Build history of the part. All positions in model axes, mm. Face numbers are marked on the shaded views. Give positions to 0.01 mm unless a question says otherwise; leave off trailing zeros. Order: outer loops, then holes, each group sorted by start corner. A loop starts at its lowest first (then second) coordinate and runs counter-clockwise, first axis right, second up. Notation, with made-up numbers: (8.25, 3.5) - (62.25, 3.5) arc R22 ccw to (62.25, 29.5) - close; hole circle Ø10 at (42, 25). An arc over 180 degrees is marked (long way). One line per item, written item: value.
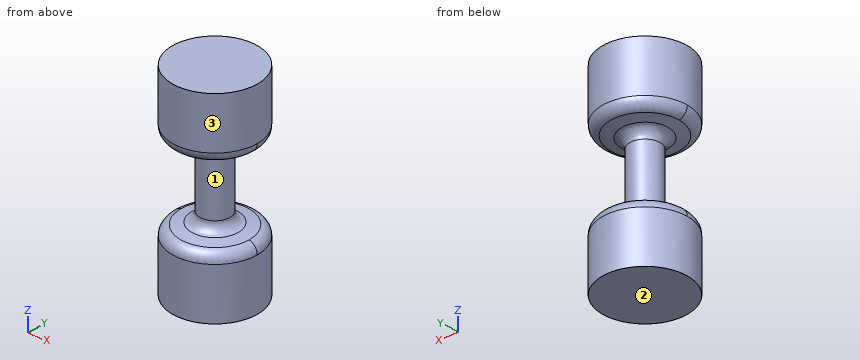
```python
from build123d import *

# Parameters (mm, degrees)
BOSS_EXTRUDE1_DEPTH      = 20
BOSS_EXTRUDE1_DEPTH_BACK = 20
SKETCH1_R                = 8.5
FILLET1_R                = 2


# Read off the part's stored shape, not the designer's step: Shell1
with BuildPart() as part:
    # Sketch1 → Boss-Extrude1 (new, two sides: drawn at the far end of the back side and taken through both)
    with BuildSketch(Plane.XY.offset(-BOSS_EXTRUDE1_DEPTH_BACK)):
        Circle(SKETCH1_R)
    extrude(amount=BOSS_EXTRUDE1_DEPTH + BOSS_EXTRUDE1_DEPTH_BACK)

    # Sketch2 → Cut-Revolve1 (revolve, cut)
    with BuildSketch(Plane(origin=(0, 0, 0), x_dir=(0, 0, -1), z_dir=(1, 0, 0)), mode=Mode.PRIVATE) as cut_revolve1_sk:
        Polygon((-8, 8.5), (8, 8.5), (7, 3), (-7, 3), align=None)
    revolve(cut_revolve1_sk.sketch.rotate(Axis((0, 0, -22), (0, 0, 1)), 90), axis=Axis((0, 0, -22), (0, 0, 1)), mode=Mode.SUBTRACT)

    # Shell1 outline → Shell1 (revolve, cut)
    with BuildSketch(Plane.XZ):
        Polygon((1, 8.669152707), (6.5, 9.669152707), (6.5, 18), (0, 18), (0, -18), (6.5, -18), (6.5, -9.669152707), (1, -8.669152707), align=None)
    revolve(axis=Axis((0, 0, 0), (0, 0, 1)), mode=Mode.SUBTRACT)

    # Fillet1
    fillet1_edges = [part.edges().sort_by_distance(p)[0] for p in [
        (3, 0, 7),
        (0, 8.5, 8),
        (0, 8.5, -8),
        (3, 0, -7),
    ]]
    fillet(fillet1_edges, radius=FILLET1_R)


solid = part.part
```
(1) Slice it at B-B, the plane x = 3.5. Count the separate pieces of the cut face and the enclosed holes in it, and give its area (3 significant figures).
Completed:
separate pieces: 2
enclosed holes: 2
area: 199 mm²
(2) Slice it at A-A, the plane z = -14. Give the cut face in (x, y).
Completed:
outline: circle Ø17 at (0, 0); hole circle Ø13 at (0, 0)
(3) Drill centre lines: line 1 (Y direction, x = 0, z = -15.5); line 2 (Z direction, x = -4.25, y = 0.75); line 3 (Y direction, x = 0, z = -1). Where is each one in solid material? Low to high.
Completed:
line 1: -8.5 to -6.5, 6.5 to 8.5
line 2: -20 to -18, -9.27 to -7.21, 7.21 to 9.27, 18 to 20
line 3: -3 to -1, 1 to 3
(4) Pin check, flat tips, straight feed: P1, Ø3, axis at y = -2, z = -0.5, coming from the -X side; P2, Ø4, axis at x = 5.5, z = 11.5, coming from the +Y side; P3, Ø6, axis at y = 4, z = 10.5, coming from the +X side. Stop position of each tip, or through.
Completed:
P1: x = -2.96
P2: y = 7.75
P3: x = 8.44
(5) Pull direction Z, two halves, no side cores. Call the marked faces 1, 2 and 3: +Z half, -Z half, draft (parallel to the pull), parting line (faces both ways), or undercut.
Completed:
face 1: undercut
face 2: -Z half
face 3: draft
